For this review, take the finished solid that the model builds, in its own axes (mm). A direction names the side the tool comes from. Round coordinates to 2 decimals unless told otherwise and drop trailing zeros. Write each loop counter-clockwise with the first axis right and the second up, starting at its lowest first coordinate (ties: lowest second). Pieces come first, ordered by that corner, then holes. Notation, with made-up numbers: (24, 71.5) -> (35, 71.5) arc R21 cw to (35, 99.5) -> close; hole circle Ø3 at (-1.5, -29.5). An arc over 180 degrees is marked (long way). Write each question's results on one line, items separated by ' | '. Start each with the question number.
Item 1: Tool access review of faces 1 (the flat face through (-35, -2, 24)), 2 (the cylindrical face through (26.01, 4.88, 32.08)), 3 (the flat face through (-27.241, 2.57, 14.567)), 4 (the flat face through (0, 7.5, 25)), 5 (the flat face through (-13, -2.5, 14)): name each direction out of +Z, -Z, +X, -X, +Y, -Y from which nothing blocks a thin tool from reaching the whole face with its end or side.
Item 2: Add section A-A (x = -15). State the section outline as (y, z) points, plus the area to 3 significant figures.
Item 3: Add section C-C (z = 30). State the section outline as (x, y) points, plus the area to 3 significant figures.
Item 4: To check wall thickness, follow line 1 along X through (y, z) = (-6.1, 16.42); line 2 along Z through (x, y) = (30, -4.75); line 3 along X through (y, z) = (-0.5, 29.5). State the ranges of each line that lie inside material, in increasing order.
Item 5: The part is to be moulded in two halves that separate along X. For faces 6 (the flat face through (0, -5, 0)), 7 (the flat face through (28, 2.6, 15.1)), 8 (the cylindrical face through (-13.648, -5.035, 12.128)), say which applies: +X half, -X half, draft (parallel to the pull), parting line (faces both ways), or undercut.
Item 6: Clearance check with flat-ended pins moving along their axes: pin 1 (5 mm diameter, centred on x = -3.5, y = 6, fed in from -Z); pin 2 (3.5 mm diameter, centred on x = 30, z = 10, fed in from +Y); pin 3 (7 mm diameter, centred on x = -30, z = 30, fed in from +Y); pin 4 (2.5 mm diameter, centred on x = -13, z = 17, fed in from -Y). State where each tip first meets the part, or that it passes through.
Item 7: Add section B-B (y = 6). State the section outline as (x, z) points, plus the area to 3 significant figures.
Item 8: Add section D-D (y = -6.5). State the section outline as (x, z) points, plus the area to 3 significant figures.
from build123d import *
from OCP.BRepFilletAPI import BRepFilletAPI_MakeChamfer

# Parameters (mm, degrees)
SKETCH1_W           = 70
SKETCH1_H           = 15
BOSS_EXTRUDE1_DEPTH = 40
SKETCH2_R           = 2.75
CUT_EXTRUDE1_DEPTH  = 56.226805086
SKETCH3_R           = 2.75
CUT_EXTRUDE2_DEPTH  = 56.226805086
CUT_EXTRUDE5_DEPTH  = 10
SKETCH4_R           = 4.5
CUT_EXTRUDE3_DEPTH  = 5
SKETCH5_R           = 4.5
CUT_EXTRUDE4_DEPTH  = 5
CHAMFER1_SIZE       = 0.3
CHAMFER2_SIZE       = 0.3
CHAMFER3_SIZE       = 0.5
CHAMFER3_SIZE2      = 2.03603283


with BuildPart() as part:
    # Sketch1 → Boss-Extrude1 (new body)
    with BuildSketch(Plane.XY):
        Rectangle(SKETCH1_W, SKETCH1_H)
    extrude(amount=BOSS_EXTRUDE1_DEPTH)

    # Sketch2 → Cut-Extrude1 (cut, through all)
    with BuildSketch(Plane(origin=(0, 7.5, 0), x_dir=(1, 0, 0), z_dir=(0, 1, 0))):
        with Locations(Location((-15, -16.42, 0), (0, 0, 270))):
            Circle(SKETCH2_R)
        with Locations(Location((15, -16.42, 0), (0, 0, 270))):
            Circle(SKETCH2_R)
    extrude(amount=-CUT_EXTRUDE1_DEPTH, mode=Mode.SUBTRACT)

    # Sketch3 → Cut-Extrude2 (cut, through all)
    with BuildSketch(Plane(origin=(0, 7.5, 0), x_dir=(1, 0, 0), z_dir=(0, 1, 0))):
        with Locations(Location((-30, -10, 0), (0, 0, 270))):
            Circle(SKETCH3_R)
        with Locations(Location((30, -10, 0), (0, 0, 90))):
            Circle(SKETCH3_R)
        with Locations(Location((-30, -30, 0), (0, 0, 270))):
            Circle(SKETCH3_R)
        with Locations(Location((30, -30, 0), (0, 0, 90))):
            Circle(SKETCH3_R)
    extrude(amount=-CUT_EXTRUDE2_DEPTH, mode=Mode.SUBTRACT)

    # Sketch7 → Cut-Extrude5 (cut)
    with BuildSketch(Plane(origin=(0, 7.5, 0), x_dir=(1, 0, 0), z_dir=(0, 1, 0))):
        Polygon((-35, 0), (35, 0), (35, -10.42), (35, -20), (21.318342095, -10.42), (-21.318342095, -10.42), (-35, -20), align=None)
    extrude(amount=-CUT_EXTRUDE5_DEPTH, mode=Mode.SUBTRACT)

    # Sketch4 → Cut-Extrude3 (cut)
    with BuildSketch(Plane(origin=(0, 7.5, 0), x_dir=(1, 0, 0), z_dir=(0, 1, 0))):
        with Locations((-30, -10)):
            Circle(SKETCH4_R)
        with Locations(Location((-30, -30, 0), (0, 0, 270))):
            Circle(SKETCH4_R)
        with Locations(Location((30, -30, 0), (0, 0, 270))):
            Circle(SKETCH4_R)
        with Locations((30, -10)):
            Circle(SKETCH4_R)
    extrude(amount=-CUT_EXTRUDE3_DEPTH, mode=Mode.SUBTRACT)

    # Sketch5 → Cut-Extrude4 (cut)
    with BuildSketch(Plane.XZ.offset(7.5)):
        with Locations(Location((-15, 16.42, 0), (0, 0, 270))):
            Circle(SKETCH5_R)
        with Locations(Location((15, 16.42, 0), (0, 0, 270))):
            Circle(SKETCH5_R)
    extrude(amount=-CUT_EXTRUDE4_DEPTH, mode=Mode.SUBTRACT)

    # Chamfer1
    chamfer1_edges = [part.edges().sort_by_distance(p)[0] for p in [
        (30, -2.5, 12.75),
        (-30, -2.5, 7.25),
        (30, 2.5, 32.75),
        (-30, 2.5, 27.25),
    ]]
    chamfer(chamfer1_edges, length=CHAMFER1_SIZE)

    # Chamfer2
    chamfer2_edges = [part.edges().sort_by_distance(p)[0] for p in [
        (30, 7.5, 25.5),
        (-30, 7.5, 25.5),
    ]]
    chamfer(chamfer2_edges, length=CHAMFER2_SIZE)

    # Chamfer3: one chamfer whose edges measure the first distance from different faces: ONE call of the kernel's chamfer builder (chamfer() names one face for all edges)
    chamfer3_edges_1 = [part.edges().sort_by_distance(p)[0] for p in [
        (-35, 0, 40),
        (-35, -5, 0),
        (35, 0, 40),
        (35, -5, 0),
    ]]
    chamfer3_edges_2 = [part.edges().sort_by_distance(p)[0] for p in [
        (-35, 2.5, 20),
    ]]
    chamfer3_side_2 = [part.faces().sort_by_distance(p)[0] for p in [
        (-35, -1.25, 25),
    ]]
    chamfer3_edges_3 = [part.edges().sort_by_distance(p)[0] for p in [
        (35, 2.5, 20),
    ]]
    chamfer3_side_3 = [part.faces().sort_by_distance(p)[0] for p in [
        (28.159171048, 2.5, 15.21),
    ]]
    chamfer3 = BRepFilletAPI_MakeChamfer(part.part.solid().wrapped)
    for e in chamfer3_edges_1:
        chamfer3.Add(CHAMFER3_SIZE, e.wrapped)
    for e in chamfer3_edges_2:
        chamfer3.Add(CHAMFER3_SIZE, CHAMFER3_SIZE2, e.wrapped, chamfer3_side_2[0].wrapped)  # the first distance lies on this face
    for e in chamfer3_edges_3:
        chamfer3.Add(CHAMFER3_SIZE, CHAMFER3_SIZE2, e.wrapped, chamfer3_side_3[0].wrapped)  # the first distance lies on this face
    add(Compound.cast(chamfer3.Shape()), mode=Mode.REPLACE)


solid = part.part
Responses:
1) face 1: +Z, -Z, -X, +Y, -Y | face 2: +Y | face 3: -Z, -X, +Y | face 4: +Z, -Z, +X, -X, +Y | face 5: -Y
2) outline: (-7.5, 0) -> (-2.5, 0) -> (-2.5, 10.42) -> (7.5, 10.42) -> (7.5, 13.67) -> (-2.5, 13.67) -> (-2.5, 11.92) -> (-7.5, 11.92) -> close; (-7.5, 20.92) -> (-2.5, 20.92) -> (-2.5, 19.17) -> (7.5, 19.17) -> (7.5, 40) -> (-7.5, 40) -> close | area: 396 mm^2
3) outline: (-35, -7.5) -> (-32.75, -7.5) -> (-32.75, 2.2) -> (-33.05, 2.5) -> (-34.5, 2.5) -> (-34.5, 7.2) -> (-34.8, 7.5) -> (-35, 7.5) -> close; (-27.25, -7.5) -> (27.25, -7.5) -> (27.25, 2.2) -> (26.95, 2.5) -> (25.5, 2.5) -> (25.5, 7.2) -> (25.2, 7.5) -> (-25.2, 7.5) -> (-25.5, 7.2) -> (-25.5, 2.5) -> (-26.95, 2.5) -> (-27.25, 2.2) -> close; (32.75, -7.5) -> (35, -7.5) -> (35, 7.5) -> (34.8, 7.5) -> (34.5, 7.2) -> (34.5, 2.5) -> (33.05, 2.5) -> (32.75, 2.2) -> close | area: 850 mm^2
4) line 1: x = -35 to -19.5, -10.5 to 10.5, 19.5 to 35 | line 2: z = 0 to 7.25, 12.75 to 27.25, 32.75 to 40 | line 3: x = -35 to -32.7, -27.3 to 27.3, 32.7 to 35
5) face 6: draft | face 7: +X half | face 8: undercut
6) pin 1: stops at z = 10.42 | pin 2: passes through | pin 3: stops at y = 2.5 | pin 4: stops at y = -2.5
7) outline: (-35, 20.5) -> (-33.33, 18.83) -> (-21.32, 10.42) -> (21.32, 10.42) -> (34.59, 19.71) -> (35, 22.04) -> (35, 39.5) -> (34.5, 40) -> (-34.5, 40) -> (-35, 39.5) -> close; hole circle Ø9 at (-30, 30); hole circle Ø5.5 at (-15, 16.42); hole circle Ø5.5 at (15, 16.42); hole circle Ø9 at (30, 30) | area: 1,760 mm^2
8) outline: (-35, 0.5) -> (-34.5, 0) -> (34.5, 0) -> (35, 0.5) -> (35, 39.5) -> (34.5, 40) -> (-34.5, 40) -> (-35, 39.5) -> close; hole circle Ø5.5 at (-30, 10); hole circle Ø5.5 at (-30, 30); hole circle Ø9 at (-15, 16.42); hole circle Ø9 at (15, 16.42); hole circle Ø5.5 at (30, 10); hole circle Ø5.5 at (30, 30) | area: 2,580 mm^2
